Answer from the drawing. Dimensions are ordinates in mm from the lowest x, y and z of the part. A direction names the side the tool comes from. Coordinates: 2 decimals unless noted, no trailing zeros. Write each loop counter-clockwise with the first axis right and the second up, starting at its lowest first coordinate (ties: lowest second). Pieces come first, ordered by that corner, then holes. Notation, with made-up numbers: (20, 6) -> (76, 6) arc R8 ccw to (76, 14) -> close; hole circle Ø10 at (-6.5, 20.5). An arc over 180 degrees is marked (long way). Answer as a JSON object with one key per item and string values. Group by question number.
(1) Find section D-D (x = 1.8). Give the vertices of the cut face in (y, z).
(2) Flat-ended cylindrical pins translate along their axes: P1, Ø13.5, axis at x = 16, y = 16.5, coming from the -Z side; P2, Ø1.6, axis at y = 8.5, z = 5.5, coming from the +X side; P3, Ø2, axis at x = 24, z = 2.5, coming from the -Y side. Find the tip coordinate at first contact, or state that the pin passes through.
(3) Find section B-B (x = 18.6). Give the vertices of the cut face in (y, z), then the cut area to 3 significant figures.
(4) Find section C-C (y = 1.8). Give the vertices of the cut face in (x, z).
(5) Straight lines are drawn through the part: L1, parallel to Y at x = 18.6, z = 2.8; L2, parallel to Z at x = 10.5, y = 14.25; L3, parallel to Z at x = 17.25, y = 3.75. For each, find the intervals that lie inside material, in ascending order.
(6) Find section A-A (z = 3.35). Give the vertices of the cut face in (x, y), then the cut area to 3 significant figures.
(7) Which of the six approach directions +Z, -Z, +X, -X, +Y, -Y give full straight-line access (tool end or side, diameter ignored) to the marked faces 1 and 2?
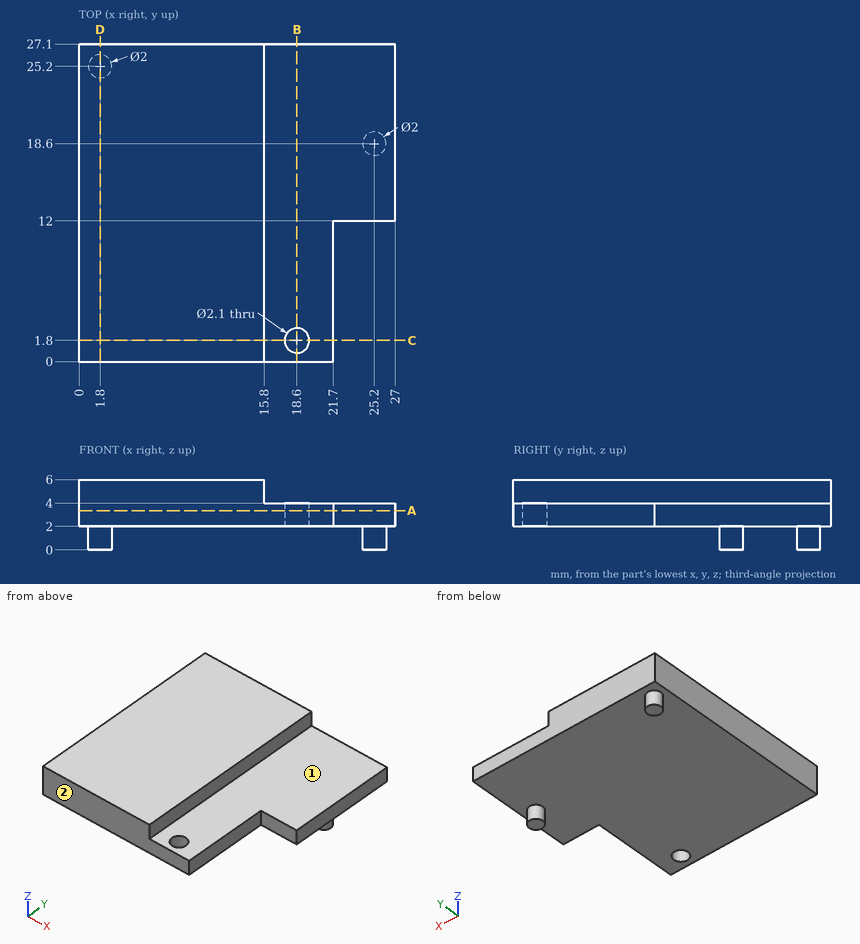
Results below:
{
 "1": {"outline": "(0, 2) -> (24.2, 2) -> (24.2, 0) -> (26.2, 0) -> (26.2, 2) -> (27.1, 2) -> (27.1, 6) -> (0, 6) -> close"},
 "2": {"P1": "stops at z = 2", "P2": "stops at x = 15.8", "P3": "stops at y = 12"},
 "3": {"outline": "(0, 2) -> (0.75, 2) -> (0.75, 4) -> (0, 4) -> close; (2.85, 2) -> (27.1, 2) -> (27.1, 4) -> (2.85, 4) -> close", "area": "50.0 mm2"},
 "4": {"outline": "(0, 2) -> (17.55, 2) -> (17.55, 4) -> (15.8, 4) -> (15.8, 6) -> (0, 6) -> close; (19.65, 2) -> (21.7, 2) -> (21.7, 4) -> (19.65, 4) -> close"},
 "5": {"L1": "y = 0 to 0.75, 2.85 to 27.1", "L2": "z = 2 to 6", "L3": "z = 2 to 4"},
 "6": {"outline": "(0, 0) -> (21.7, 0) -> (21.7, 12) -> (27, 12) -> (27, 27.1) -> (0, 27.1) -> close; hole circle Ø2.1 at (18.6, 1.8)", "area": "665 mm2"},
 "7": {"face 1": "+Z, +X, +Y, -Y", "face 2": "+Z, -Z, +X, -X, -Y"}
}
